Verification items for the finished model (mm, model axes). A direction names the side the tool comes from. Give positions to 0.01 mm unless a question says otherwise; leave off trailing zeros. Loops run counter-clockwise (first coordinate to the right, second up) from the corner with the lowest first, then second, coordinate; pieces in that order, holes last. Notation, with made-up numbers: (18, -23) -> (26, -23) arc R10 cw to (26, -10) -> close; hole circle Ø8 at (-23, 10.25). An arc over 180 degrees is marked (long way). Answer in a Markdown table with one row per item. Add a question column.
Q1. Section check B-B on x = 209.5. Enter the section's corners in (y, z).
Q2. Material ranges on probe 1 along X at (y, z) = (109, -19); probe 2 along X at (y, z) = (205, -19); probe 3 along X at (y, z) = (53.5, -4), recorded low to high.
Q3. Set-up check for faces 3 (the face through (489, 190.5, -15)), 4 (the face through (19, 304.8, -15)), 5 (the face through (469.9, 105, -9)), 6 (the face through (38.1, 276, -9)): record each of +Z, -Z, +X, -X, +Y, -Y from which the full face is reachable in a straight line by a thin tool's end or side.
Q4. Gauge pin test, flat ends, axial feed: P1, Ø5.5, axis at y = 180.5, z = -8, coming from the -X side; P2, Ø5, axis at y = 207.5, z = -25.5, coming from the -X side; P3, Ø9.5, axis at y = 234.5, z = -13, coming from the +X side. Record the tip position at first contact, or that the pin passes through.
Q5. Release check for a two-part mould opening along Y. For faces 1 (the face through (19, 57.15, -15)), 2 (the face through (38.1, 124, -9)) record: pulls with the +Y half, pulls with the -Y half, needs draft (parallel to the pull), parting line crosses it, or undercut.
```python
from build123d import *

# Parameters (mm, degrees)
F0_W      = 508
F0_H      = 361.95
F1_DEPTH  = 19.05
F2_W      = 38.1
F2_H      = 19.05
F3_DEPTH  = 38.1
F4_R      = 19.04999
F5_R      = 19.04999
F6_R      = 3.175
F7_DEPTH  = 361.951
F8_W      = 38.1
F8_H      = 38.1
F9_DEPTH  = 361.951
F10_W     = 38.1
F10_H     = 19.05
F11_DEPTH = 38.1
F12_R     = 19.04999
F13_R     = 3.175
F14_DEPTH = 342.901


# Not quite as in the source:
# - a fillet or chamfer is up to 0.001 mm smaller than in the source, because OpenCascade refuses the exact size


with BuildPart() as f1:
    # F0 (on Top) → F1 (new body)
    with BuildSketch(Plane.XY):
        with Locations((254, 180.975)):
            Rectangle(F0_W, F0_H)
    extrude(amount=F1_DEPTH)

    # F2 (on face) → F3 (join)
    with BuildSketch(Plane(origin=(0, 0, 0), x_dir=(1, 0, 0), z_dir=(0, 0, -1))):
        with Locations((19.05, -9.525)):
            Rectangle(F2_W, F2_H)
        with Locations((19.05, -47.625)):
            Rectangle(F2_W, F2_H)
        with Locations((19.05, -85.725)):
            Rectangle(F2_W, F2_H)
        with Locations((19.05, -123.825)):
            Rectangle(F2_W, F2_H)
        with Locations((19.05, -161.925)):
            Rectangle(F2_W, F2_H)
        with Locations((19.05, -200.025)):
            Rectangle(F2_W, F2_H)
        with Locations((19.05, -238.125)):
            Rectangle(F2_W, F2_H)
        with Locations((19.05, -276.225)):
            Rectangle(F2_W, F2_H)
        with Locations((19.05, -314.325)):
            Rectangle(F2_W, F2_H)
        with Locations((19.05, -352.425)):
            Rectangle(F2_W, F2_H)
        with Locations((488.95, -9.525)):
            Rectangle(F2_W, F2_H)
        with Locations((488.95, -47.625)):
            Rectangle(F2_W, F2_H)
        with Locations((488.95, -85.725)):
            Rectangle(F2_W, F2_H)
        with Locations((488.95, -123.825)):
            Rectangle(F2_W, F2_H)
        with Locations((488.95, -161.925)):
            Rectangle(F2_W, F2_H)
        with Locations((488.95, -200.025)):
            Rectangle(F2_W, F2_H)
        with Locations((488.95, -238.125)):
            Rectangle(F2_W, F2_H)
        with Locations((488.95, -276.225)):
            Rectangle(F2_W, F2_H)
        with Locations((488.95, -314.325)):
            Rectangle(F2_W, F2_H)
        with Locations((488.95, -352.425)):
            Rectangle(F2_W, F2_H)
    extrude(amount=F3_DEPTH)

    # F4 (radius 19.05 in the source; OpenCascade refuses exactly that, so slightly less here)
    f4_edges = [f1.edges().sort_by_distance(p)[0] for p in [
        (508, 9.525, -38.1),
        (469.9, 9.525, -38.1),
        (469.9, 47.625, -38.1),
        (508, 47.625, -38.1),
        (508, 85.725, -38.1),
        (469.9, 85.725, -38.1),
        (469.9, 123.825, -38.1),
        (508, 123.825, -38.1),
        (508, 161.925, -38.1),
        (469.9, 161.925, -38.1),
        (508, 200.025, -38.1),
        (469.9, 200.025, -38.1),
        (469.9, 238.125, -38.1),
        (508, 238.125, -38.1),
        (469.9, 276.225, -38.1),
        (508, 276.225, -38.1),
        (469.9, 314.325, -38.1),
        (508, 314.325, -38.1),
        (469.9, 352.425, -38.1),
        (508, 352.425, -38.1),
    ]]
    fillet(f4_edges, radius=F4_R)

    # F5 (radius 19.05 in the source; OpenCascade refuses exactly that, so slightly less here)
    f5_edges = [f1.edges().sort_by_distance(p)[0] for p in [
        (38.1, 9.525, -38.1),
        (0, 9.525, -38.1),
        (38.1, 47.625, -38.1),
        (0, 47.625, -38.1),
        (38.1, 85.725, -38.1),
        (0, 85.725, -38.1),
        (38.1, 123.825, -38.1),
        (0, 123.825, -38.1),
        (0, 161.925, -38.1),
        (38.1, 161.925, -38.1),
        (38.1, 200.025, -38.1),
        (0, 200.025, -38.1),
        (0, 238.125, -38.1),
        (38.1, 238.125, -38.1),
        (38.1, 276.225, -38.1),
        (0, 276.225, -38.1),
        (38.1, 314.325, -38.1),
        (0, 314.325, -38.1),
        (38.1, 352.425, -38.1),
        (0, 352.425, -38.1),
    ]]
    fillet(f5_edges, radius=F5_R)

    # F6 (on face) → F7 (cut, through all)
    with BuildSketch(Plane.XZ):
        with Locations((19.05, -19.05)):
            Circle(F6_R)
        with Locations((488.95, -19.05)):
            Circle(F6_R)
    extrude(amount=-F7_DEPTH, mode=Mode.SUBTRACT)

    # F8 (on face) → F9 (cut, through all)
    with BuildSketch(Plane.XZ):
        with Locations((488.95, -19.05)):
            Rectangle(F8_W, F8_H)
    extrude(amount=-F9_DEPTH, mode=Mode.SUBTRACT)

    # F10 (on face) → F11 (join)
    with BuildSketch(Plane(origin=(0, 0, 0), x_dir=(1, 0, 0), z_dir=(0, 0, -1))):
        with Locations((488.95, -28.575)):
            Rectangle(F10_W, F10_H)
        with Locations((488.95, -66.675)):
            Rectangle(F10_W, F10_H)
        with Locations((488.95, -104.775)):
            Rectangle(F10_W, F10_H)
        with Locations((488.95, -142.875)):
            Rectangle(F10_W, F10_H)
        with Locations((488.95, -180.975)):
            Rectangle(F10_W, F10_H)
        with Locations((488.95, -219.075)):
            Rectangle(F10_W, F10_H)
        with Locations((488.95, -257.175)):
            Rectangle(F10_W, F10_H)
        with Locations((488.95, -295.275)):
            Rectangle(F10_W, F10_H)
        with Locations((488.95, -333.375)):
            Rectangle(F10_W, F10_H)
    extrude(amount=F11_DEPTH)

    # F12 (radius 19.05 in the source; OpenCascade refuses exactly that, so slightly less here)
    f12_edges = [f1.edges().sort_by_distance(p)[0] for p in [
        (469.9, 28.575, -38.1),
        (508, 28.575, -38.1),
        (508, 66.675, -38.1),
        (508, 104.775, -38.1),
        (508, 142.875, -38.1),
        (508, 180.975, -38.1),
        (469.9, 66.675, -38.1),
        (469.9, 104.775, -38.1),
        (469.9, 142.875, -38.1),
        (469.9, 180.975, -38.1),
        (469.9, 219.075, -38.1),
        (469.9, 257.175, -38.1),
        (469.9, 295.275, -38.1),
        (469.9, 333.375, -38.1),
        (508, 333.375, -38.1),
        (508, 295.275, -38.1),
        (508, 219.075, -38.1),
        (508, 257.175, -38.1),
    ]]
    fillet(f12_edges, radius=F12_R)

    # F13 (on face) → F14 (cut, through all)
    with BuildSketch(Plane.XZ.offset(-19.05)):
        with Locations((488.95, -19.05)):
            Circle(F13_R)
    extrude(amount=-F14_DEPTH, mode=Mode.SUBTRACT)


solid = f1.part
```
Taken from the geometry:
| question | item | result |
|---|---|---|
| 1 | outline | (0, 0) -> (361.95, 0) -> (361.95, 19.05) -> (0, 19.05) -> close |
| 2 | probe 1 | x = 469.9 to 485.78, 492.12 to 508 |
| 2 | probe 2 | x = 0 to 15.88, 22.22 to 38.1 |
| 2 | probe 3 | x = 0 to 38.1 |
| 3 | face 3 | -Z, +X |
| 3 | face 4 | -Z, -X |
| 3 | face 5 | -Z, -X, +Y, -Y |
| 3 | face 6 | -Z, +X, +Y, -Y |
| 4 | P1 | stops at x = 469.9 |
| 4 | P2 | stops at x = 0.41 |
| 4 | P3 | stops at x = 38.1 |
| 5 | face 1 | undercut |
| 5 | face 2 | needs draft |
